Can you work these out from the model? Positions are in its coordinate system, mm. A direction names the side the tool comes from. Give positions to 0.01 mm unless a question says otherwise; leave off trailing zeros. Write each loop counter-clockwise with the first axis right and the second up, starting at its lowest first coordinate (ties: lowest second). Pieces come first, ordered by that corner, then holes.
Autodesk Inventor part; units mm, degrees
ref_plane "작업 평면1" through (21.2, 0, 0) normal (1, 0, 0) x (0, 1, 0)
ref_plane "작업 평면5" through (0, 21.2, 0) normal (0, 1, 0) x (-1, 0, 0)
ref_plane "YZ Plane" through (0, 0, 0) normal (1, 0, 0) x (0, 1, 0)
sketch "스케치1" plane through (0, 0, 0) normal (0, 0, 1) x (1, 0, 0)
  circle A0 centre (0, 0) radius 21.2
  dimension "d0" = 42.4
extrude "돌출1" add sketch "스케치1" along normal blind 45.9
sketch "스케치2" plane through (0, 0, 45.9) normal (0, 0, 1) x (1, 0, 0)
  circle A0 centre (0, 0) radius 12.5
  line L0 (-11.5, -4.899) -> (-11.5, 4.899)
  line L1 (11.5, -4.899) -> (11.5, 4.899)
  line L2 (0, 0) -> (17.5, 0) construction
  circle A1 centre (12.3744, -12.3744) radius 2
  circle A2 centre (12.3744, 12.3744) radius 2
  circle A3 centre (-12.3744, 12.3744) radius 2
  circle A4 centre (-12.3744, -12.3744) radius 2
  dimension "d5" = 360
extrude "돌출2" cut sketch "스케치2" against normal blind 6 contours A1 | A2 | A3 | A4
sketch "스케치3" plane through (0, 0, 45.9) normal (0, 0, 1) x (1, 0, 0)
  circle A0 centre (0, 0) radius 12.5
  line L0 (-11.5, -4.899) -> (-11.5, 4.899)
  line L1 (11.5, -4.899) -> (11.5, 4.899)
  line L2 (0, 0) -> (17.5, 0) construction
  circle A1 centre (12.3744, -12.3744) radius 2
  circle A2 centre (12.3744, 12.3744) radius 2
  circle A3 centre (-12.3744, 12.3744) radius 2
  circle A4 centre (-12.3744, -12.3744) radius 2
  dimension "d10" = 360
extrude "돌출3" add sketch "스케치3" along normal blind 2 contours L1 A0 L0
sketch "스케치4" plane through (0, 0, 47.9) normal (0, 0, 1) x (1, 0, 0)
  circle A0 centre (0, 0) radius 4
  dimension "d13" = 8
extrude "돌출4" cut sketch "스케치4" against normal blind 5
ref_plane "작업 평면1" through (21.2, 0, 0) normal (1, 0, 0) x (0, 1, 0)
sketch "스케치5" plane through (21.2, 0, 0) normal (1, 0, 0) x (0, 1, 0)
  line L0 (21.2, 45.9) -> (-21.2, 45.9)
  line L1 (21.2, 0) -> (-21.2, 0)
  line L2 (-4.899, 45.9) -> (4.899, 45.9)
  line L3 (0, 45.9) -> (0, 35.9)
  line L4 (0, 35.9) -> (0, 10)
  circle A0 centre (0, 10) radius 4
  circle A1 centre (0, 35.9) radius 4
  point P0 (0, 0)
  dimension "d16" = 10
  dimension "d17" = 25.9
  dimension "d18" = 8
extrude "돌출5" cut sketch "스케치5" against normal blind 0.5
ref_plane "작업 평면5" through (0, 21.2, 0) normal (0, 1, 0) x (-1, 0, 0)
sketch "스케치7" plane through (0, 21.2, 0) normal (0, 1, 0) x (-1, 0, 0)
  line L0 (0, 0) -> (0, 35.9)
  line L1 (-11.5, 45.9) -> (11.5, 45.9)
  circle A0 centre (0, 35.9) radius 4
  dimension "d28" = 35.9
  dimension "d29" = 8
extrude "돌출7" cut sketch "스케치7" against normal blind 0.5
pattern_circular "원형 패턴2" count 2 over 360 about axis through (0, 0, 0) along (0, 0, 1) of "돌출5", "돌출7"
fillet "모깎기1" radius 1 1 edges at (-21.2, 0, 0)
properties part number "gear(49ratio)"
(1) Imagine slicing it at C-C, the plane z = 35.9. Write out the boundary of the cut face in (x, y), plus the area to 3 significant figures.
Returned:
outline: (-20.82, -4) arc R21.2 ccw to (-4, -20.82) - (-4, -20.7) - (4, -20.7) - (4, -20.82) arc R21.2 ccw to (20.82, -4) - (20.7, -4) - (20.7, 4) - (20.82, 4) arc R21.2 ccw to (4, 20.82) - (4, 20.7) - (-4, 20.7) - (-4, 20.82) arc R21.2 ccw to (-20.82, 4) - (-20.7, 4) - (-20.7, -4) - close
area: 1,400 mm2
(2) If we mould it in two halves opening along Y, with no side actions, what happens to faces 6 (the face through (12, -12, 39.9)), 7 (the face through (0, 0, 0)), 8 (the face through (20.7, 0, 10)), 9 (the face through (0, 20.7, 36))? For each: +Y half, -Y half, draft (parallel to the pull), parting line (faces both ways), or undercut.
Returned:
face 6: undercut
face 7: draft
face 8: undercut
face 9: +Y half
(3) For faces 1 (the face through (0.2, -12.5, 46.9)), 2 (the face through (-0.2, 12.5, 46.9)), 3 (the face through (-0.867, -3.905, 45.435)), 4 (the face through (19.583, 8.12, 23.136)), 5 (the face through (-20.7, 0, 36)), which set-ups out of +Z, -Z, +X, -X, +Y, -Y let a thin tool reach every point of the face, with its end or its side?
Returned:
face 1: +Z, -Y
face 2: +Z, +Y
face 3: +Z
face 4: +Z, -Z
face 5: -X
(4) If I drill on L1, parallel to Z at x = 21.05, y = 0; L2, parallel to Y at x = 0.5, z = 40; L3, parallel to Z at x = -7, y = 14, over which ranges is the centre line in solid material (lowest first)?
Returned:
L1: z = 0.47 to 6, 14 to 31.9, 39.9 to 45.9
L2: y = -21.19 to 21.19
L3: z = 0 to 45.9
(5) Imagine slicing it at D-D, the plane z = 7. Write out the boundary of the cut face in (x, y), plus the area to 3 significant figures.
Returned:
outline: (-21.03, -2.65) arc R21.2 ccw to (21.03, -2.65) - (20.7, -2.65) - (20.7, 2.65) - (21.03, 2.65) arc R21.2 ccw to (-21.03, 2.65) - (-20.7, 2.65) - (-20.7, -2.65) - close
area: 1,410 mm2
(6) Will these pins go through, and if not, where does the flat tip stop? P1, Ø3, axis at x = 9, z = 30, coming from the -Y side; P2, Ø2.5, axis at x = -2, z = 36.5, coming from the +Y side; P3, Ø0.6, axis at y = 1.5, z = 47, coming from the -X side.
Returned:
P1: stops at y = -19.83
P2: stops at y = 20.7
P3: stops at x = -11.5
(7) Imagine slicing it at A-A, the plane x = 0. Write out the boundary of the cut face in (y, z), plus the area to 3 significant figures.
Returned:
outline: (-21.2, 1) arc R1 ccw to (-20.2, 0) - (20.2, 0) arc R1 ccw to (21.2, 1) - (21.2, 31.9) - (20.7, 31.9) - (20.7, 39.9) - (21.2, 39.9) - (21.2, 45.9) - (12.5, 45.9) - (12.5, 47.9) - (4, 47.9) - (4, 42.9) - (-4, 42.9) - (-4, 47.9) - (-12.5, 47.9) - (-12.5, 45.9) - (-21.2, 45.9) - (-21.2, 39.9) - (-20.7, 39.9) - (-20.7, 31.9) - (-21.2, 31.9) - close
area: 1,950 mm2
